Can you work these out from the drawing? Everything is in mm from the part's minimum corner. A direction names the side the tool comes from. Coordinates: 2 decimals unless noted, no trailing zeros. Write each loop counter-clockwise with the first axis right and the second up, starting at its lowest first coordinate (ties: lowest second). Pieces come first, ordered by that corner, then holes.
(1) Thinking about a two-plate mould opening in Z: for the marked faces 3, 4 and 5, which applies, released by +Z, released by -Z, zero draft, split by the parting line, or undercut?
(2) Imagine slicing it at C-C, the plane y = 4.75. List the corners of the cut face in (x, z) for me.
(3) Imagine slicing it at D-D, the plane x = 32. List the corners of the cut face in (y, z) for me, plus the area to 3 significant figures.
(4) For pin 1 Ø1.1 at (x, y) = (9.5, 7.5) entering from -Z; pin 2 Ø8 at (x, z) = (28, 17) entering from +Y; pin 3 Ø2.5 at (y, z) = (8, 16.5) entering from -X; pin 4 Ø1.8 at (y, z) = (8, 17.5) entering from +X, each with a flat end and sliding along its axis, tell me the tip position at first contact or that it passes through.
(5) Imagine slicing it at B-B, the plane x = 7.5. List the corners of the cut face in (y, z) for me.
(6) Which directions (+Z, -Z, +X, -X, +Y, -Y) give clear straight access to the entire face, cutting with the end or side of a thin tool? Please do the marked faces 1 and 2.
(7) Imagine slicing it at A-A, the plane z = 18. List the corners of the cut face in (x, y) for me.
(8) Please list where these lines run through material, in increasing order: probe 1 along X at (y, z) = (6.75, 23); probe 2 along Z at (x, y) = (27.5, 7.5); probe 3 along Z at (x, y) = (8, 7.5).
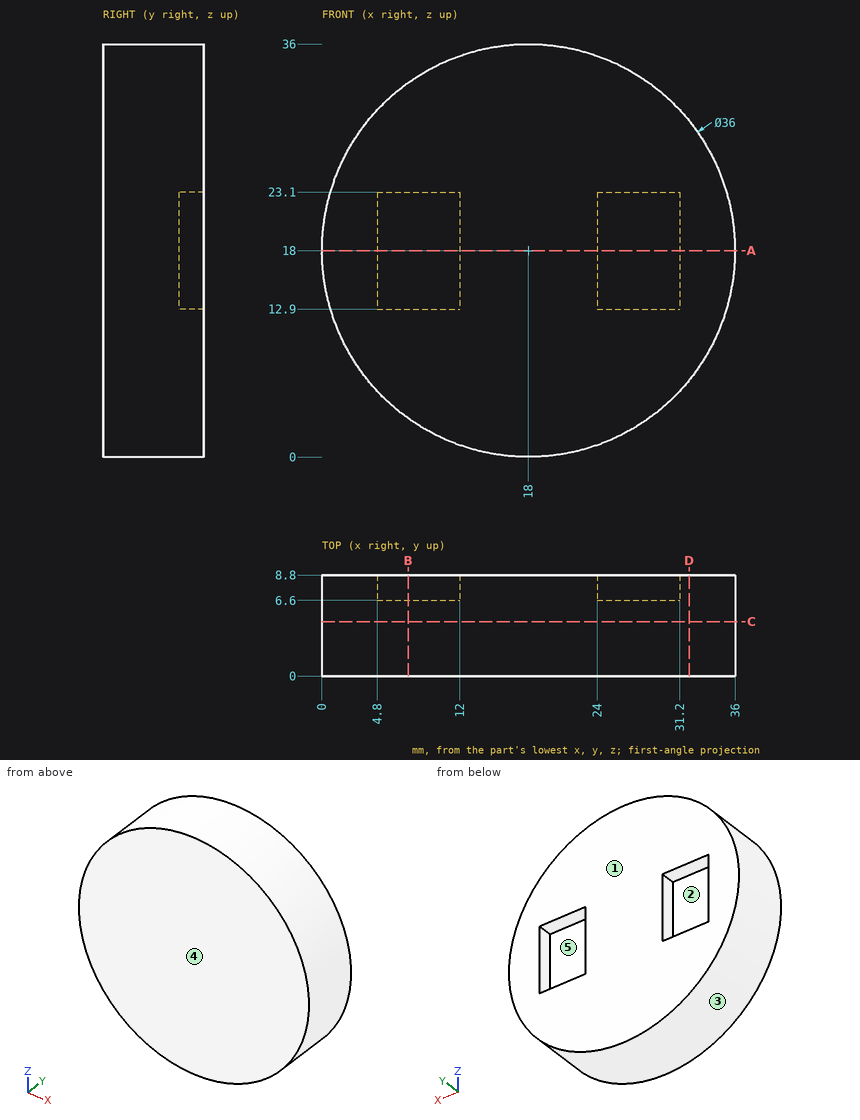
Recorded:
1. face 3: split by the parting line
1. face 4: zero draft
1. face 5: undercut
2. outline: circle Ø36 at (18, 18)
3. outline: (0, 6.69) - (8.8, 6.69) - (8.8, 29.31) - (0, 29.31) - close
3. area: 199 mm2
4. pin 1: stops at z = 1.85
4. pin 2: stops at y = 8.8
4. pin 3: stops at x = 0
4. pin 4: stops at x = 36
5. outline: (0, 3.38) - (8.8, 3.38) - (8.8, 12.9) - (6.6, 12.9) - (6.6, 23.1) - (8.8, 23.1) - (8.8, 32.62) - (0, 32.62) - close
6. face 1: +Z, -Z, +X, -X, +Y
6. face 2: +Y
7. outline: (0, 0) - (36, 0) - (36, 8.8) - (31.2, 8.8) - (31.2, 6.6) - (24, 6.6) - (24, 8.8) - (12, 8.8) - (12, 6.6) - (4.8, 6.6) - (4.8, 8.8) - (0, 8.8) - close
8. probe 1: x = 0.71 to 4.8, 12 to 24, 31.2 to 35.29
8. probe 2: z = 2.71 to 12.9, 23.1 to 33.29
8. probe 3: z = 3.03 to 12.9, 23.1 to 32.97
